Print and shaded views of the part. All mm, measured from the part's lowest x, y and z. Round coordinates to 2 decimals unless told otherwise and drop trailing zeros. Order: outer loops, then holes, each group sorted by start corner. A loop starts at its lowest first (then second) coordinate and runs counter-clockwise, first axis right, second up. Notation, with made-up numbers: (-30.5, -3) - (-12.5, -3) arc R27 ccw to (-12.5, 32) - close; hole circle Ø11 at (39, -19). An arc over 180 degrees is marked (long way). Return JSON: item names as keys, results as strings. Group by question number.
Item 1: Saw through at A-A on y = 6.25. List the corners of the cut face in (x, z), and give its area (3 significant figures).
Item 2: Saw through at D-D on y = 2. List the corners of the cut face in (x, z).
Item 3: Saw through at B-B on z = 0.55. List the corners of the cut face in (x, y) (1 decimal).
Item 4: Probe probe 1 along Y at (x, z) = (76.2, 0.55) (1 decimal); probe 2 along X at (y, z) = (8, 1.3); probe 3 along X at (y, z) = (8.75, 0.35) (1 decimal). List the from-to ranges inside material, lowest first.
Item 5: Saw through at C-C on x = 78.5. List the corners of the cut face in (y, z) (1 decimal).
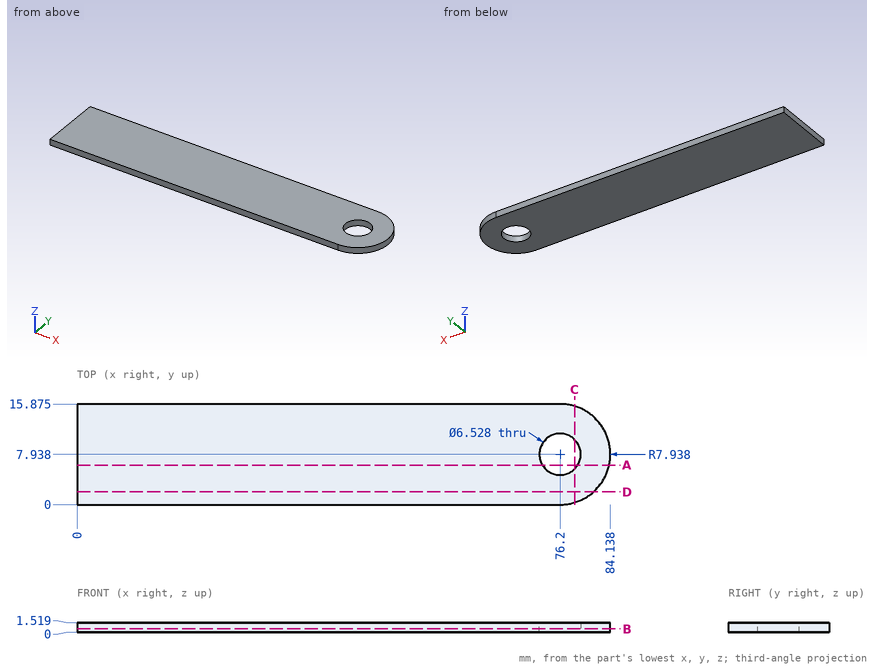
Filled in:
{
 "1": {"outline": "(0, 0) - (73.41, 0) - (73.41, 1.52) - (0, 1.52) - close; (78.99, 0) - (83.96, 0) - (83.96, 1.52) - (78.99, 1.52) - close", "area": "119 mm^2"},
 "2": {"outline": "(0, 0) - (81.47, 0) - (81.47, 1.52) - (0, 1.52) - close"},
 "3": {"outline": "(0, 0) - (76.2, 0) arc R7.9 ccw to (76.2, 15.9) - (0, 15.9) - close; hole circle Ø6.5 at (76.2, 7.9)"},
 "4": {"probe 1": "y = 0 to 4.7, 11.2 to 15.9", "probe 2": "x = 0 to 72.94, 79.46 to 84.14", "probe 3": "x = 0 to 73, 79.4 to 84.1"},
 "5": {"outline": "(0.3, 0) - (5.6, 0) - (5.6, 1.5) - (0.3, 1.5) - close; (10.3, 0) - (15.5, 0) - (15.5, 1.5) - (10.3, 1.5) - close"}
}
